The model under review builds one solid part; all positions refer to its coordinate system, in mm. A direction names the side the tool comes from. Coordinates: 2 decimals unless noted, no trailing zeros. Loops run counter-clockwise (first coordinate to the right, second up) from the corner with the lowest first, then second, coordinate; pieces in that order, holes last. Notation, with made-up numbers: M 10.25,52.5 L 58.25,52.5 A13 cw 58.25,69.5 Z; hole C 79.25,72 d7. An arc over 180 degrees is marked long. Return JSON: item names as keys, results as strings.
```python
from build123d import *

# Parameters (mm, degrees)
SKETCH2_W          = 2.5
SKETCH2_H          = 3.5
CUT_EXTRUDE1_DEPTH = 3.5
FILLET1_R          = 0.5
CUT_EXTRUDE2_DEPTH = 0.5


with BuildPart() as part:
    # Sketch1 → Revolve1 (revolve)
    with BuildSketch(Plane.XY, mode=Mode.PRIVATE) as revolve1_sk:
        Polygon((0, 7.25), (5, 7.25), (5, 1.25), (8, 1.25), (8, 0), (0, 0), align=None)
    revolve(revolve1_sk.sketch.rotate(Axis((0, 7.25, 0), (0, -1, 0)), 180), axis=Axis((0, 7.25, 0), (0, -1, 0)))

    # Sketch2 → Cut-Extrude1 (cut)
    with BuildSketch(Plane.XZ):
        Rectangle(SKETCH2_W, SKETCH2_H)
    extrude(amount=-CUT_EXTRUDE1_DEPTH, mode=Mode.SUBTRACT)

    # Fillet1
    fillet1_edges = [part.edges().sort_by_distance(p)[0] for p in [
        (5, 7.25, 0),
    ]]
    fillet(fillet1_edges, radius=FILLET1_R)

    # Sketch3 → Cut-Extrude2 (cut)
    with BuildSketch(Plane(origin=(0, 7.25, 0), x_dir=(1, 0, 0), z_dir=(0, 1, 0))):
        Polygon((0.338942308, 3.153846154), (1.461538462, 3.153846154), (1.461538462, -0.769230769), (2, -0.769230769), (2, -1.769230769), (1.461538462, -1.769230769), (1.461538462, -3), (0.384615385, -3), (0.384615385, -1.769230769), (-2.153846154, -1.769230769), (-2.153846154, -0.679086538), align=None)
        Polygon((0.384615385, -0.769230769), (0.384615385, 1.272836538), (-0.943509615, -0.769230769), align=None, mode=Mode.SUBTRACT)
    extrude(amount=-CUT_EXTRUDE2_DEPTH, mode=Mode.SUBTRACT)


solid = part.part
```
1. Add section C-C on x = 0. Give the boundary of the cut face in (y, z), plus the area to 3 significant figures.
Check values:
{"outline": "M 0,-8 L 1.25,-8 L 1.25,-5 L 6.75,-5 A0.5 ccw 7.25,-4.5 L 7.25,-2.63 L 6.75,-2.63 L 6.75,-0.68 L 7.25,-0.68 L 7.25,0.77 L 6.75,0.77 L 6.75,1.77 L 7.25,1.77 L 7.25,4.5 A0.5 ccw 6.75,5 L 1.25,5 L 1.25,8 L 0,8 L 0,1.75 L 3.5,1.75 L 3.5,-1.75 L 0,-1.75 Z", "area": "66.2 mm²"}
2. Machinability: for faces 4 (the face through (0, 7.25, 2)), 5 (the face through (5, 4, 0)), 6 (the face through (1.25, 2, 0)), which of the approach directions +Z, -Z, +X, -X, +Y, -Y give a long, thin tool a straight path to every point of the face, cutting with its end or side? Answer none if there is none.
Check values:
{"face 4": "+Z, -Z, +X, -X, +Y", "face 5": "+Y", "face 6": "-Y"}
3. Add section A-A on y = 0.5. Give the boundary of the cut face in (x, z).
Check values:
{"outline": "C 0,0 d16; hole M -1.25,-1.75 L 1.25,-1.75 L 1.25,1.75 L -1.25,1.75 Z"}
4. Insertion check: pin 1 Ø1.2 at (x, y) = (0, 2.5) entering from -Z; pin 2 Ø1.5 at (x, y) = (2, 1) entering from -Z; pin 3 Ø0.6 at (x, y) = (1, 7) entering from -Z. Each pin has a flat end and moves straight along its axis. Give the tip position at first contact, or say it passes through.
Check values:
{"pin 1": "z = -5", "pin 2": "z = -7.9", "pin 3": "z = -4.94"}
5. Add section D-D on y = 6.5. Give the boundary of the cut face in (x, z).
Check values:
{"outline": "C 0,0 d10"}
6. Add section B-B on z = 0. Give the boundary of the cut face in (x, y).
Check values:
{"outline": "M -8,0 L -1.25,0 L -1.25,3.5 L 1.25,3.5 L 1.25,0 L 8,0 L 8,1.25 L 5,1.25 L 5,6.75 A0.5 ccw 4.5,7.25 L 1.46,7.25 L 1.46,6.75 L 0.38,6.75 L 0.38,7.25 L -0.44,7.25 L -0.44,6.75 L -1.71,6.75 L -1.71,7.25 L -4.5,7.25 A0.5 ccw -5,6.75 L -5,1.25 L -8,1.25 Z"}
7. The part is to be moulded in two halves that separate along Z. For faces 1 (the face through (0, 7.25, 0)), 2 (the face through (1.73, 0.62, 7.81)), 3 (the face through (0, 2, 1.75)), say which applies: released by +Z, released by -Z, zero draft, split by the parting line, or undercut.
Check values:
{"face 1": "zero draft", "face 2": "split by the parting line", "face 3": "undercut"}
8. To check wall thickness, follow line 1 (Y direction, x = -3.5, z = -5.25); line 2 (Z direction, x = 0, y = 3); line 3 (X direction, y = 3, z = -1.25). State the ranges of each line that lie inside material, in increasing order.
Check values:
{"line 1": "0 to 1.25", "line 2": "-5 to -1.75, 1.75 to 5", "line 3": "-4.84 to -1.25, 1.25 to 4.84"}
